```python
from build123d import *

# Parameters (mm, degrees)
BOSS_EXTRU_1_DEPTH                  = 4.5
BOSS_EXTRU_2_START                  = 22.2
ESQUISSE2_R                         = 7
BOSS_EXTRU_2_DEPTH                  = 22.2
DIAM_TRE_DU_PER_AGE_4_2_4_2_1_D     = 4.2
DIAM_TRE_DU_PER_AGE_4_2_4_2_1_DEPTH = 10
DIAM_TRE_DU_PER_AGE_6_0_6_1_D       = 6


with BuildPart() as part:
    # Esquisse1 → Boss.-Extru.1 (new body)
    with BuildSketch(Plane(origin=(0, 0, 0), x_dir=(-1, 0, 0), z_dir=(0, 0, -1))):
        with BuildLine():
            Line((0, 7), (-30, 7))
            ThreePointArc((-30, 7), (-37, 0), (-30, -7))
            Line((-30, -7), (0, -7))
            ThreePointArc((0, -7), (7, 0), (0, 7))
        make_face()
    extrude(amount=-BOSS_EXTRU_1_DEPTH)

    # Esquisse2 → Boss.-Extru.2 (add)
    with BuildSketch(Plane(origin=(0, 0, 0), x_dir=(-1, 0, 0), z_dir=(0, 0, -1)).offset(BOSS_EXTRU_2_START)):
        with Locations((-30, 0)):
            Circle(ESQUISSE2_R)
    extrude(amount=-BOSS_EXTRU_2_DEPTH)

    # Diamètre du perçage Ø4.2 (4.2)1
    with Locations(Plane(origin=(0, 0, -22.2), x_dir=(-1, 0, 0), z_dir=(0, 0, -1))):
        with Locations((-30, 0)):
            Hole(DIAM_TRE_DU_PER_AGE_4_2_4_2_1_D / 2, depth=DIAM_TRE_DU_PER_AGE_4_2_4_2_1_DEPTH)

    # Diamètre du perçage Ø6.0 (6)1 (through all)
    with Locations(Plane(origin=(0, 0, 0), x_dir=(-1, 0, 0), z_dir=(0, 0, -1))):
        with Locations((0, 0)):
            Hole(DIAM_TRE_DU_PER_AGE_6_0_6_1_D / 2)


solid = part.part
```
Can you work these out from the model? Positions are in its coordinate system, mm. A direction names the side the tool comes from. Give positions to 0.01 mm unless a question says otherwise; leave off trailing zeros. Write each loop counter-clockwise with the first axis right and the second up, starting at its lowest first coordinate (ties: lowest second). Pieces come first, ordered by that corner, then holes. Notation, with made-up numbers: (64, -18.5) -> (76, -18.5) arc R28 ccw to (76, 18.5) -> close; hole circle Ø9 at (75, -16.75). An arc over 180 degrees is marked (long way). One line per item, written item: value.
Q1. Which directions (+Z, -Z, +X, -X, +Y, -Y) give clear straight access to the entire face, cutting with the end or side of a thin tool? Please do faces 1 (the face through (15, -7, 2)), 2 (the face through (30, 0, -12.2)).
Results found:
face 1: +Z, -Z, +X, -X, -Y
face 2: -Z
Q2. We'd pull the mould along X, two halves only. Please class faces 3 (the face through (-3, 0, 2)), 4 (the face through (-7, 0, 2)), 5 (the face through (37, 0, -9)), 6 (the face through (27.9, 0.09, -17.13)): +X half, -X half, draft (parallel to the pull), parting line (faces both ways), or undercut.
Results found:
face 3: undercut
face 4: -X half
face 5: parting line
face 6: undercut
Q3. Imagine slicing it at B-B on z = -17.5. Please give me the cut outline in (x, y), and give its area (3 significant figures).
Results found:
outline: circle Ø14 at (30, 0); hole circle Ø4.2 at (30, 0)
area: 140 mm^2
Q4. Imagine slicing it at C-C on x = 28.5. Please give me the cut outline in (y, z), and give its area (3 significant figures).
Results found:
outline: (-7, 0) -> (-6.84, 0) -> (-6.84, -22.2) -> (-1.47, -22.2) -> (-1.47, -12.2) -> (1.47, -12.2) -> (1.47, -22.2) -> (6.84, -22.2) -> (6.84, 0) -> (7, 0) -> (7, 4.5) -> (-7, 4.5) -> close
area: 337 mm^2
Q5. Imagine slicing it at A-A on y = 0. Please give me the cut outline in (x, z).
Results found:
outline: (-7, 0) -> (-3, 0) -> (-3, 4.5) -> (-7, 4.5) -> close; (3, 0) -> (23, 0) -> (23, -22.2) -> (27.9, -22.2) -> (27.9, -12.2) -> (32.1, -12.2) -> (32.1, -22.2) -> (37, -22.2) -> (37, 4.5) -> (3, 4.5) -> close
Q6. Imagine slicing it at D-D on z = -5. Please give me the cut outline in (x, y), and give its area (3 significant figures).
Results found:
outline: circle Ø14 at (30, 0)
area: 154 mm^2
Q7. Please list where these lines run through material, in increasing order: line 1 (Y direction, x = 30, z = -18); line 2 (Y direction, x = 0, z = 2.85); line 3 (Z direction, x = 27, y = -6.5). Write a range as [from, to].
Results found:
line 1: y = [-7, -2.1], [2.1, 7]
line 2: y = [-7, -3], [3, 7]
line 3: z = [0, 4.5]
Q8. For P1, Ø3, axis at x = -1.5, y = -4.5, coming from the -Z side; P2, Ø4, axis at x = 23.5, z = -16, coming from the -Y side; P3, Ø4, axis at x = 30, y = 0, coming from the -Z side, each with a flat end and sliding along its axis, tell me the tip position at first contact or that it passes through.
Results found:
P1: stops at z = 0
P2: stops at y = -5.36
P3: stops at z = -12.2
